Could you check a few things on this model? Use its own coordinates, in mm. Face numbers are marked on the shaded views. A direction names the side the tool comes from. Round coordinates to 2 decimals unless told otherwise and drop trailing zeros. Write each loop counter-clockwise with the first axis right and the second up, starting at its lowest first coordinate (ties: lowest second). Pieces come first, ordered by that corner, then holes. Notation, with made-up numbers: (22.25, 88.25) -> (33.25, 88.25) arc R22 ccw to (33.25, 118.25) -> close; hole circle Ø6 at (88.25, 10). An arc over 180 degrees is marked (long way). One line per question, with ' | ' between items. Start each with the question number.
1. Imagine slicing it at B-B, the plane z = 50.8. List the corners of the cut face in (x, y) for me (3 decimals), and give its area (3 significant figures).
2. Imagine slicing it at A-A, the plane y = 533.4. List the corners of the cut face in (x, z) for me (3 decimals), and give its area (3 significant figures).
3. If I drill on line 1 along Y through (x, z) = (4, 50); line 2 along X through (y, z) = (76, 2); line 3 along Z through (x, y) = (2.25, 533.4) (3 decimals), over which ranges is the centre line in solid material (lowest first)? Write a range as [from, to].
4. Imagine slicing it at D-D, the plane z = 90. List the corners of the cut face in (x, y) for me, and give its area (3 significant figures).
5. Imagine slicing it at C-C, the plane x = 49.5. List the corners of the cut face in (y, z) for me, and give its area (3 significant figures).
6. For the marked faces 1 and 2, which set-ups out of +Z, -Z, +X, -X, +Y, -Y let a thin tool reach every point of the face, with its end or its side?
7. For pin 1 Ø25 at (y, z) = (304.8, 50.8) entering from -X; pin 2 Ø25 at (y, z) = (533.4, 50.8) entering from +X; pin 3 Ø8 at (x, y) = (85, 452.5) entering from +Z, each with a flat end and sliding along its axis, tell me the tip position at first contact or that it passes through.
from build123d import *

# Parameters (mm, degrees)
F1_DEPTH = 609.6
F2_R     = 9.525
F3_DEPTH = 25.4
F4_R     = 9.525
F5_DEPTH = 25.4


with BuildPart() as f1:
    # F0 (on Front) → F1 (new body)
    with BuildSketch(Plane.XZ):
        Polygon((0, 101.6), (0, 0), (101.6, 0), (101.6, 6.35), (6.35, 6.35), (6.35, 101.6), align=None)
    extrude(amount=-F1_DEPTH)

    # F2 (on face) → F3 (cut)
    with BuildSketch(Plane(origin=(0, 0, 0), x_dir=(0, -1, 0), z_dir=(-1, 0, 0))):
        with Locations((-533.4, 50.8)):
            Circle(F2_R)
        with Locations((-304.8, 50.8)):
            Circle(F2_R)
        with Locations((-76.2, 50.8)):
            Circle(F2_R)
    extrude(amount=-F3_DEPTH, mode=Mode.SUBTRACT)

    # F4 (on face) → F5 (cut)
    with BuildSketch(Plane(origin=(0, 0, 0), x_dir=(1, 0, 0), z_dir=(0, 0, -1))):
        with Locations((50.8, -533.4)):
            Circle(F4_R)
        with Locations((50.8, -304.8)):
            Circle(F4_R)
        with Locations((50.8, -76.2)):
            Circle(F4_R)
    extrude(amount=-F5_DEPTH, mode=Mode.SUBTRACT)


solid = f1.part
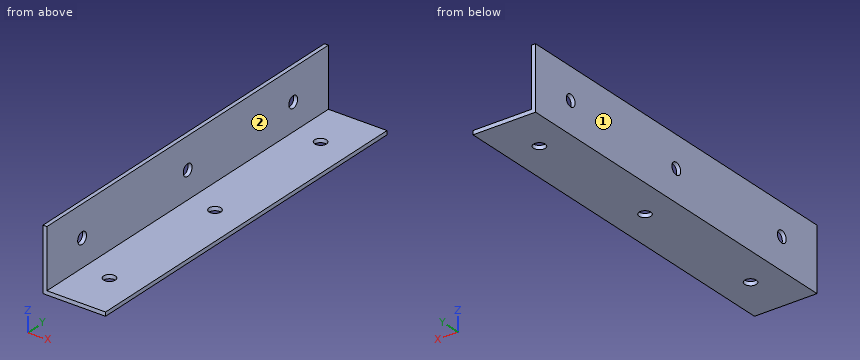
Geometry results:
1) outline: (0, 0) -> (6.35, 0) -> (6.35, 66.675) -> (0, 66.675) -> close; (0, 85.725) -> (6.35, 85.725) -> (6.35, 295.275) -> (0, 295.275) -> close; (0, 314.325) -> (6.35, 314.325) -> (6.35, 523.875) -> (0, 523.875) -> close; (0, 542.925) -> (6.35, 542.925) -> (6.35, 609.6) -> (0, 609.6) -> close | area: 3,510 mm2
2) outline: (0, 0) -> (41.275, 0) -> (41.275, 6.35) -> (6.35, 6.35) -> (6.35, 41.275) -> (0, 41.275) -> close; (0, 60.325) -> (6.35, 60.325) -> (6.35, 101.6) -> (0, 101.6) -> close; (60.325, 0) -> (101.6, 0) -> (101.6, 6.35) -> (60.325, 6.35) -> close | area: 1,010 mm2
3) line 1: y = [0, 66.71], [85.69, 295.31], [314.29, 523.91], [542.89, 609.6] | line 2: x = [0, 41.28], [60.32, 101.6] | line 3: z = [0, 41.275], [60.325, 101.6]
4) outline: (0, 0) -> (6.35, 0) -> (6.35, 609.6) -> (0, 609.6) -> close | area: 3,870 mm2
5) outline: (0, 0) -> (66.76, 0) -> (66.76, 6.35) -> (0, 6.35) -> close; (85.64, 0) -> (295.36, 0) -> (295.36, 6.35) -> (85.64, 6.35) -> close; (314.24, 0) -> (523.96, 0) -> (523.96, 6.35) -> (314.24, 6.35) -> close; (542.84, 0) -> (609.6, 0) -> (609.6, 6.35) -> (542.84, 6.35) -> close | area: 3,510 mm2
6) face 1: +Z, -Z, -X, +Y, -Y | face 2: +Z, +X, +Y, -Y
7) pin 1: stops at x = 0 | pin 2: stops at x = 6.35 | pin 3: stops at z = 6.35
